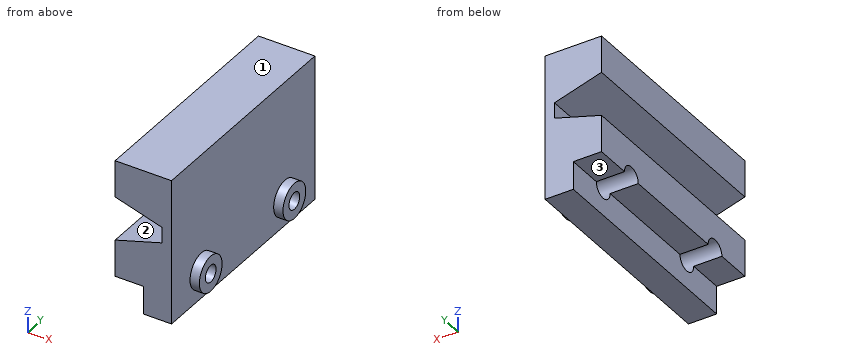
from build123d import *

# Parameters (mm, degrees)
BOSS_EXTRUDE1_DEPTH = 24
SKETCH7_W           = 3.015
SKETCH7_H           = 24
BOSS_EXTRUDE3_DEPTH = 3
SKETCH3_R           = 1.9
SKETCH3_R_2         = 0.9
BOSS_EXTRUDE2_DEPTH = 1
SKETCH4_R           = 1.15
CUT_EXTRUDE2_DEPTH  = 23
CUT_EXTRUDE3_DEPTH  = 30


with BuildPart() as part:
    # Sketch1 → Boss-Extrude1 (new body)
    with BuildSketch(Plane(origin=(0, 0, 0), x_dir=(1, 0, 0), z_dir=(0, 1, 0))):
        Polygon((0.758759529, 5.315), (5, 5.315), (5, -7.215), (1.398203198, -7.215), (-1.03, -7.215), (-1.03, -1.785), (4, -1.785), (4, -0.115), (-1.03, -0.115), (-1.03, 5.315), align=None)
    extrude(amount=BOSS_EXTRUDE1_DEPTH)

    # Sketch7 → Boss-Extrude3 (add)
    with BuildSketch(Plane(origin=(0, 0, -5.315), x_dir=(-1, 0, 0), z_dir=(0, 0, -1))):
        with Locations((-3.4925, 12)):
            Rectangle(SKETCH7_W, SKETCH7_H)
    extrude(amount=BOSS_EXTRUDE3_DEPTH)

    # Sketch3 → Boss-Extrude2 (add)
    with BuildSketch(Plane(origin=(5, 0, 0), x_dir=(0, 0, -1), z_dir=(1, 0, 0))):
        with Locations((5.315, 19)):
            Circle(SKETCH3_R)
        with Locations((5.315, 19)):
            Circle(SKETCH3_R_2, mode=Mode.SUBTRACT)
        with Locations((5.315, 5)):
            Circle(SKETCH3_R)
        with Locations((5.315, 5)):
            Circle(SKETCH3_R_2, mode=Mode.SUBTRACT)
    extrude(amount=BOSS_EXTRUDE2_DEPTH)

    # Sketch4 → Cut-Extrude2 (cut)
    with BuildSketch(Plane(origin=(5, 0, 0), x_dir=(0, 0, -1), z_dir=(1, 0, 0))):
        with Locations((5.315, 19)):
            Circle(SKETCH4_R)
        with Locations((5.315, 5)):
            Circle(SKETCH4_R)
    extrude(amount=-CUT_EXTRUDE2_DEPTH, mode=Mode.SUBTRACT)

    # Sketch6 → Cut-Extrude3 (cut)
    with BuildSketch(Plane(origin=(0, 24, 0), x_dir=(1, 0, 0), z_dir=(0, 1, 0))):
        Polygon((-1.03, -0.115), (4, -0.115), (-1.03, 1.385), align=None)
        Polygon((4, -1.785), (-1.03, -1.785), (-1.03, -3.285), align=None)
    extrude(amount=-CUT_EXTRUDE3_DEPTH, mode=Mode.SUBTRACT)


solid = part.part
Verification items for the finished model (mm, model axes). Face numbers are marked on the shaded views. A direction names the side the tool comes from. Give positions to 0.01 mm unless a question says otherwise; leave off trailing zeros. Loops run counter-clockwise (first coordinate to the right, second up) from the corner with the lowest first, then second, coordinate; pieces in that order, holes last.
1) Sectioned sample at D-D, the plane x = 1.5. Enter the section's corners in (y, z) (3 decimals), then the cut area to 3 significant figures.
2) Set-up check for the marked faces 1, 2 and 3: record each of +Z, -Z, +X, -X, +Y, -Y from which the full face is reachable in a straight line by a thin tool's end or side.
3) Thickness scan on line 1 along X through (y, z) = (2.75, -2.25); line 2 along Z through (x, y) = (0.25, 3.25) (3 decimals); line 3 along Z through (x, y) = (1, 11) (3 decimals). Record the ranges inside material, lowest first.
4) Sectioned sample at C-C, the plane y = 16. Enter the section's corners in (x, z) (3 decimals), then the cut area to 3 significant figures.
5) Depth check by flat-ended pin: pin 1 Ø1.6 at (y, z) = (5, -5.315) entering from -X; pin 2 Ø0.9 at (x, y) = (0, 22.5) entering from -Z (3 decimals); pin 3 Ø4.5 at (y, z) = (10.5, 3.5) entering from +X; pin 4 Ø2.5 at (y, z) = (11.5, -7.5) entering from -X (3 decimals). Enter the tip coordinate at first touch or a pass-through.
6) Sectioned sample at A-A, the plane y = 19. Enter the section's corners in (x, z) (3 decimals), then the cut area to 3 significant figures.
7) Sectioned sample at B-B, the plane x = 3.25. Enter the section's corners in (y, z) (3 decimals), then the cut area to 3 significant figures.
Answers:
1. outline: (0, -5.315) - (3.85, -5.315) arc R1.15 cw to (6.15, -5.315) - (17.85, -5.315) arc R1.15 cw to (20.15, -5.315) - (24, -5.315) - (24, -0.631) - (0, -0.631) - close; (0, 2.531) - (24, 2.531) - (24, 7.215) - (0, 7.215) - close
1. area: 221 mm2
2. face 1: +Z, +X, -X, +Y, -Y
2. face 2: -X, +Y, -Y
2. face 3: -Z, -X, +Y, -Y
3. line 1: x = -1.03 to 5
3. line 2: z = -5.315 to -1.003, 2.903 to 7.215
3. line 3: z = -5.315 to -0.78, 2.68 to 7.215
4. outline: (-1.03, -5.315) - (1.985, -5.315) - (1.985, -8.315) - (5, -8.315) - (5, 7.215) - (-1.03, 7.215) - (-1.03, 3.285) - (4, 1.785) - (4, 0.115) - (-1.03, -1.385) - close
4. area: 68.7 mm2
5. pin 1: passes through
5. pin 2: stops at z = -5.315
5. pin 3: stops at x = 5
5. pin 4: stops at x = 1.985
6. outline: (-1.03, -4.165) - (5, -4.165) - (5, -4.415) - (6, -4.415) - (6, -3.415) - (5, -3.415) - (5, 7.215) - (-1.03, 7.215) - (-1.03, 3.285) - (4, 1.785) - (4, 0.115) - (-1.03, -1.385) - close; (1.985, -8.315) - (5, -8.315) - (5, -7.215) - (6, -7.215) - (6, -6.215) - (5, -6.215) - (5, -6.465) - (1.985, -6.465) - close
6. area: 60.3 mm2
7. outline: (0, -8.315) - (24, -8.315) - (24, -0.109) - (0, -0.109) - close; (0, 2.009) - (24, 2.009) - (24, 7.215) - (0, 7.215) - close; hole circle Ø2.3 at (5, -5.315); hole circle Ø2.3 at (19, -5.315)
7. area: 314 mm2
